from build123d import *

# Parameters (mm, degrees)
SKETCH013_W     = 41
SKETCH013_H     = 10
SKETCH013_R     = 1.45
PAD009_DEPTH    = 5
SKETCH014_R     = 1.6
POCKET002_DEPTH = 7
SKETCH015_W     = 2
SKETCH015_H     = 6
POCKET003_DEPTH = 8


with BuildPart() as part:
    # Sketch013 → Pad009 (new body, symmetric)
    with BuildSketch(Plane.XY):
        with Locations((20.5, 0)):
            Rectangle(SKETCH013_W, SKETCH013_H)
        with Locations((33.5, 0)):
            Circle(SKETCH013_R, mode=Mode.SUBTRACT)
        with Locations((8.5, 0)):
            Circle(SKETCH013_R, mode=Mode.SUBTRACT)
    extrude(amount=PAD009_DEPTH, both=True)

    # Sketch014 → Pocket002 (cut)
    with BuildSketch(Plane.YZ):
        Circle(SKETCH014_R)
    extrude(amount=POCKET002_DEPTH, mode=Mode.SUBTRACT)

    # Sketch015 → Pocket003 (cut)
    with BuildSketch(Plane.XY.offset(5)):
        with Locations((4.5, 0)):
            Rectangle(SKETCH015_W, SKETCH015_H)
    extrude(amount=-POCKET003_DEPTH, mode=Mode.SUBTRACT)


solid = part.part
Work out the finished part from the listing and answer in its coordinate system (mm). A direction names the side the tool comes from. Round coordinates to 2 decimals unless told otherwise and drop trailing zeros. Order: outer loops, then holes, each group sorted by start corner. A loop starts at its lowest first (then second) coordinate and runs counter-clockwise, first axis right, second up. Notation, with made-up numbers: M 86.25,89 L 111.25,89 A13 cw 111.25,96 Z; hole C -12.5,-8 d9. An arc over 180 degrees is marked long. Put each result on its own line as item: value. Start each with the question number.
Q1. A tool of negligible diameter and unlimited length cuts with its end or side. For faces 1 (the flat face through (4, -3, 1)), 2 (the cylindrical face through (34.839, -0.555, -0.07)), 3 (the cylindrical face through (6.24, -1.27, -0.97)), from which of +Z, -Z, +X, -X, +Y, -Y can it reach the whole face along a straight path? Write none if from no direction.
Q2. Section A-A, the plane y = 0 is taken. Write down the section's boundary in (x, z), and give its area (3 significant figures).
Q3. Section D-D, the plane x = 6 is taken. Write down the section's boundary in (y, z).
Q4. A flat-ended cylindrical pin translates along its axis: pin 1 (0.6 mm diameter, centred on x = 5, y = -1, fed in from +Z). Find the tip coordinate at first contact, or state that the pin passes through.
Q5. Straight lines are drawn through the part: L1, parallel to X at y = -1, z = -3.5; L2, parallel to X at y = 2.5, z = 0.25; L3, parallel to Y at x = 8.5, z = -2. For each, find the intervals that lie inside material, in ascending order. Write a range as [from, to].
Q6. For a pull along X with two mould halves and no side action, classify faces 4 (the flat face through (5.5, 0, 2)), 5 (the flat face through (41, 0, 0)), 6 (the flat face through (20, 0, 5)), 7 (the flat face through (3.5, 0, 2)) as pulls with the +X half, pulls with the -X half, needs draft (parallel to the pull), parting line crosses it, or undercut.
Q7. Section C-C, the plane z = 0 is taken. Write down the section's boundary in (x, y), and give its area (3 significant figures).
Q8. Section B-B, the plane x = 33.5 is taken. Write down the section's boundary in (y, z), and give its area (3 significant figures).
Findings below:
1. face 1: +Z
1. face 2: +Z, -Z
1. face 3: -X
2. outline: M 0,-5 L 7.05,-5 L 7.05,5 L 5.5,5 L 5.5,1.6 L 7,1.6 L 7,-1.6 L 5.5,-1.6 L 5.5,-3 L 3.5,-3 L 3.5,-1.6 L 0,-1.6 Z; M 0,1.6 L 3.5,1.6 L 3.5,5 L 0,5 Z; M 9.95,-5 L 32.05,-5 L 32.05,5 L 9.95,5 Z; M 34.95,-5 L 41,-5 L 41,5 L 34.95,5 Z
2. area: 320 mm^2
3. outline: M -5,-5 L 5,-5 L 5,5 L -5,5 Z; hole C 0,0 d3.2
4. pin 1: stops at z = -3
5. L1: x = [0, 7.45], [9.55, 32.45], [34.55, 41]
5. L2: x = [0, 3.5], [5.5, 41]
5. L3: y = [-5, -1.45], [1.45, 5]
6. face 4: undercut
6. face 5: pulls with the +X half
6. face 6: needs draft
6. face 7: undercut
7. outline: M 0,-5 L 41,-5 L 41,5 L 0,5 L 0,1.6 L 3.5,1.6 L 3.5,3 L 5.5,3 L 5.5,1.6 L 7,1.6 L 7,-1.6 L 5.5,-1.6 L 5.5,-3 L 3.5,-3 L 3.5,-1.6 L 0,-1.6 Z; hole C 8.5,0 d2.9; hole C 33.5,0 d2.9
7. area: 369 mm^2
8. outline: M -5,-5 L -1.45,-5 L -1.45,5 L -5,5 Z; M 1.45,-5 L 5,-5 L 5,5 L 1.45,5 Z
8. area: 71.0 mm^2
